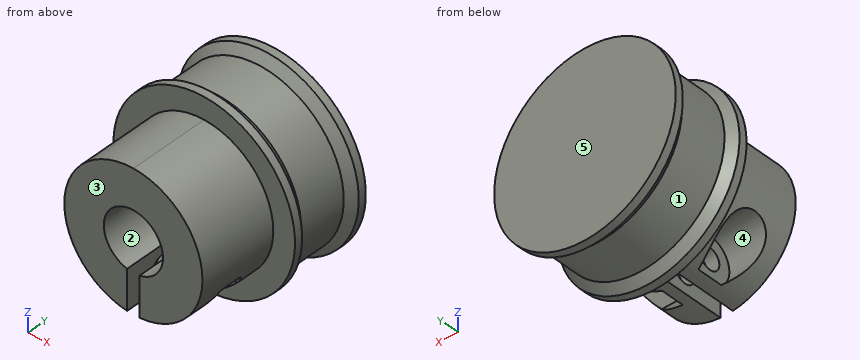
```python
from build123d import *

# Parameters (mm, degrees)
SKETCH1_R                           = 11.1125
BOSS_EXTRUDE1_DEPTH                 = 12.7
CUT_EXTRUDE1_START                  = -12.7
SKETCH2_R                           = 4
CUT_EXTRUDE1_DEPTH                  = 12.7
CUT_EXTRUDE2_START                  = -12.7
SKETCH3_R                           = 4.7625
CUT_EXTRUDE2_DEPTH                  = 12.7
CUT_EXTRUDE3_REACH                  = 31.869
CUT_EXTRUDE4_DEPTH                  = 4
CUT_EXTRUDE4_DIRECTION_2_REACH      = 26.756
CUT_EXTRUDE4_DIRECTION_2_END_RADIUS = 11.1125
M3_CLEARANCE_HOLE1_D                = 3.4
CUT_EXTRUDE5_REACH                  = 23.999
SKETCH9_R                           = 3.5
SKETCH10_R                          = 14.605
BOSS_EXTRUDE2_DEPTH                 = 12.7
CUT_EXTRUDE6_START                  = -2.54
SKETCH11_R                          = 14.605
SKETCH11_R_2                        = 13.335
CUT_EXTRUDE6_DEPTH                  = 7.62
CHAMFER1_SIZE                       = 1.27


# Read off the part's stored shape, not the designer's step: Split1
with BuildPart() as part:
    # Sketch1 → Boss-Extrude1 (new, symmetric)
    with BuildSketch(Plane(origin=(0, 0, 0), x_dir=(1, 0, 0), z_dir=(0, 1, 0))):
        with Locations(Location((0, 0, 0), (0, 0, 270))):
            Circle(SKETCH1_R)
    extrude(amount=BOSS_EXTRUDE1_DEPTH, both=True)

    # Sketch2 → Cut-Extrude1 (cut)
    with BuildSketch(Plane(origin=(0, 12.7, 0), x_dir=(1, 0, 0), z_dir=(0, 1, 0)).offset(CUT_EXTRUDE1_START)):
        with Locations(Location((0, 0, 0), (0, 0, 270))):
            Circle(SKETCH2_R)
    extrude(amount=CUT_EXTRUDE1_DEPTH, mode=Mode.SUBTRACT)

    # Sketch3 → Cut-Extrude2 (cut)
    with BuildSketch(Plane.XZ.offset(12.7).offset(CUT_EXTRUDE2_START)):
        with Locations(Location((0, 0, 0), (0, 0, 270))):
            Circle(SKETCH3_R)
    extrude(amount=CUT_EXTRUDE2_DEPTH, mode=Mode.SUBTRACT)

    # Sketch4 → Cut-Extrude3 (cut, up to next)
    with BuildSketch(Plane(origin=(0, 12.7, 0), x_dir=(1, 0, 0), z_dir=(0, 1, 0)), mode=Mode.PRIVATE) as cut_extrude3_sk1:
        with BuildLine():
            Line((-1, 3.872983346), (-1, 11.067414163))
            ThreePointArc((-1, 11.067414163), (0, 11.1125), (1, 11.067414163))
            Line((1, 11.067414163), (1, 3.872983346))
            ThreePointArc((1, 3.872983346), (0, 4), (-1, 3.872983346))
        make_face()
    cut_extrude3_tool1 = extrude(cut_extrude3_sk1.sketch, amount=-CUT_EXTRUDE3_REACH, mode=Mode.PRIVATE) & part.part
    add(cut_extrude3_tool1.solids().sort_by_distance((0, 12.7, -7.527621))[0], mode=Mode.SUBTRACT)

    # Sketch5 → Cut-Extrude4 (cut)
    with BuildSketch(Plane(origin=(7, 0, 0), x_dir=(0, 0, -1), z_dir=(1, 0, 0))):
        Polygon((7.86187193, 2.885898385), (10.86187193, 4.617949192), (10.86187193, 8.082050808), (7.86187193, 9.814101615), (4.86187193, 8.082050808), (4.86187193, 4.617949192), align=None)
        Polygon((7.86187193, -9.814101615), (10.86187193, -8.082050808), (10.86187193, -4.617949192), (7.86187193, -2.885898385), (4.86187193, -4.617949192), (4.86187193, -8.082050808), align=None)
    extrude(amount=-CUT_EXTRUDE4_DEPTH, mode=Mode.SUBTRACT)

    # Cut-Extrude4 direction 2: up to this cylinder (the profile starts inside it)
    cut_extrude4_direction_2_end = Plane(origin=(0, 0, 0), z_dir=(0, -1, 0)) * Cylinder(CUT_EXTRUDE4_DIRECTION_2_END_RADIUS, 89.437, mode=Mode.PRIVATE)
    # Sketch5 → Cut-Extrude4 direction 2 (cut, up to the surface)
    with BuildSketch(Plane(origin=(7, 0, 0), x_dir=(0, 0, -1), z_dir=(1, 0, 0)), mode=Mode.PRIVATE) as cut_extrude4_direction_2_sk1:
        Polygon((7.86187193, 2.885898385), (10.86187193, 4.617949192), (10.86187193, 8.082050808), (7.86187193, 9.814101615), (4.86187193, 8.082050808), (4.86187193, 4.617949192), align=None)
    cut_extrude4_direction_2_tool1 = extrude(cut_extrude4_direction_2_sk1.sketch, amount=CUT_EXTRUDE4_DIRECTION_2_REACH, mode=Mode.PRIVATE) & cut_extrude4_direction_2_end
    add(cut_extrude4_direction_2_tool1.solids().sort_by_distance((7, 6.35, -7.861872))[0], mode=Mode.SUBTRACT)
    # Sketch5 → Cut-Extrude4 direction 2 (cut, up to the surface)
    with BuildSketch(Plane(origin=(7, 0, 0), x_dir=(0, 0, -1), z_dir=(1, 0, 0)), mode=Mode.PRIVATE) as cut_extrude4_direction_2_sk2:
        Polygon((7.86187193, -9.814101615), (10.86187193, -8.082050808), (10.86187193, -4.617949192), (7.86187193, -2.885898385), (4.86187193, -4.617949192), (4.86187193, -8.082050808), align=None)
    cut_extrude4_direction_2_tool2 = extrude(cut_extrude4_direction_2_sk2.sketch, amount=CUT_EXTRUDE4_DIRECTION_2_REACH, mode=Mode.PRIVATE) & cut_extrude4_direction_2_end
    add(cut_extrude4_direction_2_tool2.solids().sort_by_distance((7, -6.35, -7.861872))[0], mode=Mode.SUBTRACT)

    # M3 Clearance Hole1 (through all)
    with Locations(Plane(origin=(3, 0, 0), x_dir=(0, 0, -1), z_dir=(1, 0, 0))):
        with Locations((7.86187193, 6.35), (7.86187193, -6.35)):
            Hole(M3_CLEARANCE_HOLE1_D / 2)

    # Sketch9 → Cut-Extrude5 (cut, up to next)
    with BuildSketch(Plane(origin=(-3, 0, 0), x_dir=(0, 0, -1), z_dir=(1, 0, 0)), mode=Mode.PRIVATE) as cut_extrude5_sk1:
        with Locations((7.86187193, 6.35)):
            Circle(SKETCH9_R)
    cut_extrude5_tool1 = extrude(cut_extrude5_sk1.sketch, amount=-CUT_EXTRUDE5_REACH, mode=Mode.PRIVATE) & part.part
    # Sketch9 → Cut-Extrude5 (cut, up to next)
    with BuildSketch(Plane(origin=(-3, 0, 0), x_dir=(0, 0, -1), z_dir=(1, 0, 0)), mode=Mode.PRIVATE) as cut_extrude5_sk2:
        with Locations((7.86187193, -6.35)):
            Circle(SKETCH9_R)
    cut_extrude5_tool2 = extrude(cut_extrude5_sk2.sketch, amount=-CUT_EXTRUDE5_REACH, mode=Mode.PRIVATE) & part.part
    add(cut_extrude5_tool1.solids().sort_by_distance((-3, 6.35, -7.861872))[0], mode=Mode.SUBTRACT)
    add(cut_extrude5_tool2.solids().sort_by_distance((-3, -6.35, -7.861872))[0], mode=Mode.SUBTRACT)


with BuildPart() as body_2:
    # Split1: the piece on the far side of the plane
    add(part.part)
    split(bisect_by=Plane(origin=(0, 0, 0), x_dir=(1, 0, 0), z_dir=(0, 1, 0)), keep=Keep.BOTTOM)

    # Sketch10 → Boss-Extrude2 (add)
    with BuildSketch(Plane(origin=(0, 0, 0), x_dir=(1, 0, 0), z_dir=(0, 1, 0))):
        with Locations(Location((0, 0, 0), (0, 0, 270))):
            Circle(SKETCH10_R)
    extrude(amount=BOSS_EXTRUDE2_DEPTH)

    # Sketch11 → Cut-Extrude6 (cut)
    with BuildSketch(Plane(origin=(0, 12.7, 0), x_dir=(1, 0, 0), z_dir=(0, 1, 0)).offset(CUT_EXTRUDE6_START)):
        with Locations(Location((0, 0, 0), (0, 0, 270))):
            Circle(SKETCH11_R)
        with Locations(Location((0, 0, 0), (0, 0, 270))):
            Circle(SKETCH11_R_2, mode=Mode.SUBTRACT)
    extrude(amount=-CUT_EXTRUDE6_DEPTH, mode=Mode.SUBTRACT)

    # Chamfer1
    chamfer1_edges = [body_2.edges().sort_by_distance(p)[0] for p in [
        (0, 10.16, -14.605),
        (0, 2.54, -14.605),
    ]]
    chamfer(chamfer1_edges, length=CHAMFER1_SIZE - 0.0001)  # a hair under: the kernel refuses the full size


with BuildPart() as part_1:
    add(part.part)

    # Split1
    split(bisect_by=Plane(origin=(0, 0, 0), x_dir=(1, 0, 0), z_dir=(0, 1, 0)), keep=Keep.TOP)


solid = body_2.part
```
Read the model definition and answer for the solid it produces. Units are mm, in the model's axes. Face numbers are marked on the shaded views. A direction names the side the tool comes from. Coordinates: 2 decimals unless noted, no trailing zeros. Loops run counter-clockwise (first coordinate to the right, second up) from the corner with the lowest first, then second, coordinate; pieces in that order, holes last. Notation, with made-up numbers: (48, 30.5) -> (57, 30.5) arc R22 cw to (57, 41.5) -> close; hole circle Ø6 at (12.5, -19). An arc over 180 degrees is marked (long way). Return JSON: item names as keys, results as strings.
Item 1: For the marked faces 4 and 5, determine the directions among +Z, -Z, +X, -X, +Y, -Y from which every point of the face is accessible in a straight line to the end or side of a thin tool.
Answers:
{"face 4": "-X", "face 5": "+Z, -Z, +X, -X, +Y"}
Item 2: Find section A-A (y = -6.35). Determine the outline of the cut face in (x, z) (1 decimal), plus the area to 3 significant figures.
Answers:
{"outline": "(-10.2, -4.4) -> (-3, -4.4) -> (-3, -6.2) -> (-1, -6.2) -> (-1, -4.7) arc R4.8 cw (long way) to (1, -4.7) -> (1, -6.2) -> (3, -6.2) -> (3, -4.9) -> (10, -4.9) arc R11.1 ccw (long way) to start; (-3, -10.7) arc R11.1 ccw to (-1, -11.1) -> (-1, -9.6) -> (-3, -9.6) -> close; (1, -11.1) arc R11.1 ccw to (3, -10.7) -> (3, -9.6) -> (1, -9.6) -> close", "area": "234 mm2"}
Item 3: For a pull along Y with two mould halves and no side action, classify the marked faces 1, 2 and 3 as +Y half, -Y half, draft (parallel to the pull), parting line (faces both ways), or undercut.
Answers:
{"face 1": "undercut", "face 2": "draft", "face 3": "-Y half"}
Item 4: Find the intervals of material crossed by probe 1 along X at (y, z) = (-5.5, -5.25); probe 2 along X at (y, z) = (-1.5, 0); probe 3 along Y at (x, z) = (-11, -4.75), in increasing order.
Answers:
{"probe 1": "x = -3 to -1, 1 to 3", "probe 2": "x = -11.11 to -4.76, 4.76 to 11.11", "probe 3": "y = 0 to 12.7"}
Item 5: Find section C-C (y = 4.25). Determine the outline of the cut face in (x, z) (3 decimals).
Answers:
{"outline": "circle Ø26.67 at (0, 0)"}
Item 6: Flat-ended cylindrical pins translate along their axes: P1, Ø4, axis at y = -6.35, z = -7.86, coming from the -X side; P2, Ø10, axis at x = 4, y = -7.5, coming from the -Z side; P3, Ø1, axis at x = 6.5, y = -6, coming from the -Z side. Find the tip coordinate at first contact, or state that the pin passes through.
Answers:
{"P1": "stops at x = -3", "P2": "stops at z = -11.07", "P3": "stops at z = -4.86"}
